from build123d import *

# Parameters (mm, degrees)
SKETCH_1_W          = 105
SKETCH_1_H          = 75
SKETCH_1_R          = 2
EXTRUDE_1_DEPTH     = 3
SKETCH_3_R          = 2
CUT_EXTRUDE_2_DEPTH = 30.8
SKETCH_6_R          = 2
CUT_EXTRUDE_4_DEPTH = 15
FILLET_1_R          = 4
SKETCH_7_W          = 10
SKETCH_7_H          = 75
EXTRUDE_2_DEPTH     = 3
FILLET_2_R          = 4
CUT_EXTRUDE_START   = -3
SKETCH_8_R          = 2
CUT_EXTRUDE_5_DEPTH = 3
CUT_EXTRUDE_6_DEPTH = 10
FILLET_3_R          = 6
CUT_EXTRUDE_7_DEPTH = 10
FILLET_4_R          = 4


with BuildPart() as part:
    # Sketch 1 → Extrude 1 (new body)
    with BuildSketch(Plane(origin=(0, 0, 0), x_dir=(1, 0, 0), z_dir=(0, 1, 0))):
        Rectangle(SKETCH_1_W, SKETCH_1_H)
        with Locations(Location((48, 33, 0), (0, 0, 270))):
            Circle(SKETCH_1_R, mode=Mode.SUBTRACT)
        with Locations(Location((-48, 33, 0), (0, 0, 270))):
            Circle(SKETCH_1_R, mode=Mode.SUBTRACT)
        with Locations(Location((-48, -33, 0), (0, 0, 270))):
            Circle(SKETCH_1_R, mode=Mode.SUBTRACT)
        with Locations(Location((48, -33, 0), (0, 0, 270))):
            Circle(SKETCH_1_R, mode=Mode.SUBTRACT)
    extrude(amount=EXTRUDE_1_DEPTH)

    # Sketch 3 → Cut-Extrude 2 (cut)
    with BuildSketch(Plane(origin=(0, 3, 0), x_dir=(1, 0, 0), z_dir=(0, 1, 0))):
        with Locations(Location((-37.99, 24, 0), (0, 0, 270))):
            Circle(SKETCH_3_R)
    extrude(amount=-CUT_EXTRUDE_2_DEPTH, mode=Mode.SUBTRACT)

    # Sketch 6 → Cut-Extrude 4 (cut)
    with BuildSketch(Plane(origin=(0, 3, 0), x_dir=(1, 0, 0), z_dir=(0, 1, 0))):
        with Locations(Location((-37.99, -24, 0), (0, 0, 270))):
            Circle(SKETCH_6_R)
        with Locations(Location((12.51, 8.5, 0), (0, 0, 270))):
            Circle(SKETCH_6_R)
        with Locations(Location((12.51, -19.5, 0), (0, 0, 270))):
            Circle(SKETCH_6_R)
    extrude(amount=-CUT_EXTRUDE_4_DEPTH, mode=Mode.SUBTRACT)

    # Fillet 1
    fillet_1_edges = [part.edges().sort_by_distance(p)[0] for p in [
        (-52.5, 1.5, 37.5),
        (-52.5, 1.5, -37.5),
    ]]
    fillet(fillet_1_edges, radius=FILLET_1_R)

    # Sketch 7 → Extrude 2 (add)
    with BuildSketch(Plane(origin=(0, 0, 0), x_dir=(1, 0, 0), z_dir=(0, 1, 0))):
        with Locations((57.5, 0)):
            Rectangle(SKETCH_7_W, SKETCH_7_H)
    extrude(amount=EXTRUDE_2_DEPTH)

    # Fillet 2
    fillet_2_edges = [part.edges().sort_by_distance(p)[0] for p in [
        (62.5, 1.5, 37.5),
        (62.5, 1.5, -37.5),
    ]]
    fillet(fillet_2_edges, radius=FILLET_2_R)

    # Sketch 8 → Cut-Extrude 5 (cut)
    with BuildSketch(Plane(origin=(0, 3, 0), x_dir=(1, 0, 0), z_dir=(0, 1, 0)).offset(CUT_EXTRUDE_START)):
        with Locations(Location((29, -33, 0), (0, 0, 270))):
            Circle(SKETCH_8_R)
        with Locations(Location((29, 33, 0), (0, 0, 270))):
            Circle(SKETCH_8_R)
        with Locations(Location((48, -33, 0), (0, 0, 270))):
            Circle(SKETCH_8_R)
        with Locations(Location((48, 33, 0), (0, 0, 270))):
            Circle(SKETCH_8_R)
    extrude(amount=CUT_EXTRUDE_5_DEPTH, mode=Mode.SUBTRACT)

    # Sketch 9 → Cut-Extrude 6 (cut)
    with BuildSketch(Plane(origin=(0, 3, 0), x_dir=(1, 0, 0), z_dir=(0, 1, 0))):
        Polygon((-52.5, 29.5), (-42.5, 19.5), (-42.5, -19.5), (-52.5, -29.5), align=None)
        Polygon((-43.5, -37.5), (-33.5, -27.5), (11.5, -27.5), (21.5, -37.5), align=None)
        Polygon((-43.5, 37.5), (-33.5, 27.5), (11.5, 27.5), (21.5, 37.5), align=None)
    extrude(amount=-CUT_EXTRUDE_6_DEPTH, mode=Mode.SUBTRACT)

    # Fillet 3
    fillet_3_edges = [part.edges().sort_by_distance(p)[0] for p in [
        (21.5, 1.5, 37.5),
        (-43.5, 1.5, 37.5),
        (-52.5, 1.5, 29.5),
        (-52.5, 1.5, -29.5),
        (-43.5, 1.5, -37.5),
        (21.5, 1.5, -37.5),
        (11.5, 1.5, -27.5),
        (-33.5, 1.5, -27.5),
        (-33.5, 1.5, 27.5),
        (11.5, 1.5, 27.5),
        (-42.5, 1.5, -19.5),
        (-42.5, 1.5, 19.5),
    ]]
    fillet(fillet_3_edges, radius=FILLET_3_R)

    # Sketch 10 → Cut-Extrude 7 (cut)
    with BuildSketch(Plane(origin=(0, 3, 0), x_dir=(1, 0, 0), z_dir=(0, 1, 0))):
        Polygon((32, -37.5), (34.886751346, -32.5), (42.113248654, -32.5), (45, -37.5), align=None)
        Polygon((32, 37.5), (34.886751346, 32.5), (42.113248654, 32.5), (45, 37.5), align=None)
    extrude(amount=-CUT_EXTRUDE_7_DEPTH, mode=Mode.SUBTRACT)

    # Fillet 4
    fillet_4_edges = [part.edges().sort_by_distance(p)[0] for p in [
        (45, 1.5, 37.5),
        (32, 1.5, 37.5),
        (34.886751346, 1.5, 32.5),
        (42.113248654, 1.5, 32.5),
        (32, 1.5, -37.5),
        (45, 1.5, -37.5),
        (42.113248654, 1.5, -32.5),
        (34.886751346, 1.5, -32.5),
    ]]
    fillet(fillet_4_edges, radius=FILLET_4_R)


solid = part.part
Input: part model. Units: mm. Frame: model coordinates. A direction names the side the tool comes from. Give positions to 0.01 mm unless a question says otherwise; leave off trailing zeros. Order: outer loops, then holes, each group sorted by start corner. A loop starts at its lowest first (then second) coordinate and runs counter-clockwise, first axis right, second up. Notation, with made-up numbers: M -35.75,23 L -7.75,23 A21 ccw -7.75,30 Z; hole C 16.5,16.25 d3. An arc over 180 degrees is marked long. Answer as a JSON object with one key per item and string values.
1. First-contact query: P1, Ø3, axis at x = -48, z = 33, coming from the +Y side; P2, Ø1.5, axis at y = 0.5, z = 26, coming from the -X side; P3, Ø1.3, axis at x = 38.5, y = 1, coming from the -Z side; P4, Ø0.8, axis at x = 38, y = 1, coming from the +Z side. Flat tips, straight axial feed; report the tip coordinate or a pass-through.
Result sheet:
{"P1": "through", "P2": "x = -49.75", "P3": "z = -32.5", "P4": "z = 32.5"}
2. Cut plane D-D, the plane x = -11.5. Output: boundary loops of the cut face in (y, z).
Result sheet:
{"outline": "M 0,-27.5 L 3,-27.5 L 3,27.5 L 0,27.5 Z"}
3. Reachability of faces 1 (the flat face through (38, 2, -32.5)), 2 (the cylindrical face through (-42.944, 1.479, -19.28)), 3 (the cylindrical face through (13.862, 1.521, 18.026)), 4 (the flat face through (17, 3, -1)), 5 (the cylindrical face through (45.335, 1.479, 36.979)) from +Z, -Z, +X, -X, +Y, -Y: full face, straight path, thin tool, end or side. Return the list, or none.
Result sheet:
{"face 1": "-Z, +Y, -Y", "face 2": "-X, +Y, -Y", "face 3": "+Y, -Y", "face 4": "+Z, -Z, +X, -X, +Y", "face 5": "+Z, +Y, -Y"}
4. Ray query, line 1 (X direction, y = 1.5, z = -8.5); line 2 (X direction, y = 1.35, z = 33); line 3 (Z direction, x = 47, y = 0.35). Return the intervals inside material, ascending. Write a range as [from, to].
Result sheet:
{"line 1": "[-42.5, 10.51], [14.51, 62.5]", "line 2": "[-52.5, -50], [-46, -39], [17, 27], [31, 35.26], [41.74, 46], [50, 62.5]", "line 3": "[-37.49, -34.73], [-31.27, 31.27], [34.73, 37.49]"}
5. Cut plane C-C, the plane y = 2.15. State how many separate pieces and enclosed holes the cut face has, and give its area (3 significant figures).
Result sheet:
{"separate pieces": "1", "enclosed holes": "10", "area": "6,790 mm²"}
6. Pull-direction query (Z, two-part tool) for faces 6 (the cylindrical face through (61.297, 1.521, -36.359)), 7 (the cylindrical face through (61.297, 1.521, 36.359)), 8 (the cylindrical face through (46.226, 1.479, 33.923)); classes: +Z half, -Z half, draft (parallel to the pull), parting line (faces both ways), or undercut.
Result sheet:
{"face 6": "-Z half", "face 7": "+Z half", "face 8": "undercut"}
7. Cut plane A-A, the plane x = -37.99. Output: boundary loops of the cut face in (y, z).
Result sheet:
{"outline": "M 0,-31.99 L 3,-31.99 L 3,-26 L 0,-26 Z; M 0,-22 L 3,-22 L 3,22 L 0,22 Z; M 0,26 L 3,26 L 3,31.99 L 0,31.99 Z"}
8. Cut plane B-B, the plane z = -8.5. Output: boundary loops of the cut face in (x, y).
Result sheet:
{"outline": "M -42.5,0 L 10.51,0 L 10.51,3 L -42.5,3 Z; M 14.51,0 L 62.5,0 L 62.5,3 L 14.51,3 Z"}
